from build123d import *

# Parameters (mm, degrees)
BOSS_EXTRUDE1_DEPTH     = 17.78
FILLET1_R               = 2
FILLET2_R               = 3
CUT_EXTRUDE5_DEPTH      = 34.999094106
CUT_EXTRUDE6_DEPTH      = 3
CUT_EXTRUDE7_DEPTH      = 3
CUT_EXTRUDE7_DEPTH_BACK = 1.5
BOSS_EXTRUDE2_DEPTH     = 8


with BuildPart() as part:
    # Sketch1 → Boss-Extrude1 (new body)
    with BuildSketch(Plane.XY):
        Polygon((0, 3), (0, 0), (7.3, 0), (7.3, 10), (13.3, 10), (19.3, 10), (19.3, 0), (26.6, 0), (26.6, 3), (20.8, 3), (20.8, 11.5), (5.8, 11.5), (5.8, 3), align=None)
    extrude(amount=-BOSS_EXTRUDE1_DEPTH)

    # Fillet1
    fillet1_edges = [part.edges().sort_by_distance(p)[0] for p in [
        (5.8, 11.5, -8.89),
        (20.8, 11.5, -8.89),
    ]]
    fillet(fillet1_edges, radius=FILLET1_R)

    # Fillet2
    fillet2_edges = [part.edges().sort_by_distance(p)[0] for p in [
        (5.8, 3, -8.89),
        (20.8, 3, -8.89),
    ]]
    fillet(fillet2_edges, radius=FILLET2_R)

    # Sketch2 → Cut-Extrude5 (cut, through all)
    with BuildSketch(Plane(origin=(0, 0, 0), x_dir=(1, 0, 0), z_dir=(0, 1, 0))):
        with BuildLine():
            Line((0, 17.78), (0, 4.65))
            ThreePointArc((0, 4.65), (1.361953467, 7.938046533), (4.65, 9.3))
            Line((4.65, 9.3), (4.65, 17.78))
            Line((4.65, 17.78), (0, 17.78))
        make_face()
        with BuildLine():
            Line((0, 4.65), (0, 0))
            Line((0, 0), (4.65, 0))
            ThreePointArc((4.65, 0), (1.361953467, 1.361953467), (0, 4.65))
        make_face()
        with BuildLine():
            ThreePointArc((21.95, 9.3), (25.238046535, 7.93804653), (26.6, 4.649999993))
            Line((26.6, 4.649999993), (26.6, 17.78))
            Line((26.6, 17.78), (21.95, 17.78))
            Line((21.95, 17.78), (21.95, 9.3))
        make_face()
        with BuildLine():
            Line((21.95, 0), (26.6, 0))
            Line((26.6, 0), (26.6, 4.649999993))
            ThreePointArc((26.6, 4.649999993), (25.23804653, 1.361953465), (21.95, 0))
        make_face()
    extrude(amount=CUT_EXTRUDE5_DEPTH, mode=Mode.SUBTRACT)

    # Sketch3 → Cut-Extrude6 (cut)
    with BuildSketch(Plane.XZ):
        with BuildLine():
            Line((7.3, -6.649999971), (7.3, -2.649999971))
            Line((7.3, -2.649999971), (5.8, -2.649999971))
            Line((5.8, -2.649999971), (5.8, -3.449999971))
            Line((5.8, -3.449999971), (4.6, -3.449999971))
            ThreePointArc((4.6, -3.449999971), (3.4, -4.649999971), (4.6, -5.849999971))
            Line((4.6, -5.849999971), (5.8, -5.849999971))
            Line((5.8, -5.849999971), (5.8, -6.649999971))
            Line((5.8, -6.649999971), (7.3, -6.649999971))
        make_face()
        with BuildLine():
            Line((20.8, -5.849999971), (22, -5.849999971))
            ThreePointArc((22, -5.849999971), (23.2, -4.649999971), (22, -3.449999971))
            Line((22, -3.449999971), (20.8, -3.449999971))
            Line((20.8, -3.449999971), (20.8, -2.649999971))
            Line((20.8, -2.649999971), (19.3, -2.649999971))
            Line((19.3, -2.649999971), (19.3, -6.649999971))
            Line((19.3, -6.649999971), (20.8, -6.649999971))
            Line((20.8, -6.649999971), (20.8, -5.849999971))
        make_face()
    extrude(amount=-CUT_EXTRUDE6_DEPTH, mode=Mode.SUBTRACT)

    # Sketch4 → Cut-Extrude7 (cut, two sides: drawn at the far end of the back side and taken through both)
    with BuildSketch(Plane(origin=(0, 3, 0), x_dir=(1, 0, 0), z_dir=(0, 1, 0)).offset(-CUT_EXTRUDE7_DEPTH_BACK)):
        Polygon((2.8, 3.189230456), (2.8, 6.110769486), (2.434936491, 5.899999971), (2.434936491, 3.399999971), align=None)
        Polygon((4.6, 2.149999971), (4.6, 4.649999971), (4.6, 7.149999971), (2.8, 6.110769486), (2.8, 3.189230456), align=None)
        Polygon((5.8, 2.842820294), (4.6, 2.149999971), (4.6, 4.649999971), (4.6, 7.149999971), (5.8, 6.457179648), align=None)
        Polygon((22, 2.149999971), (22, 4.649999971), (22, 7.149999971), (20.8, 6.457179648), (20.8, 2.842820294), align=None)
        Polygon((24.165063509, 5.899999971), (24.165063509, 3.399999971), (22, 2.149999971), (22, 4.649999971), (22, 7.149999971), align=None)
    extrude(amount=CUT_EXTRUDE7_DEPTH + CUT_EXTRUDE7_DEPTH_BACK, mode=Mode.SUBTRACT)

    # Sketch5 → Boss-Extrude2 (add)
    with BuildSketch(Plane(origin=(0, 0, 0), x_dir=(-1, 0, 0), z_dir=(0, 0, -1))):
        with BuildLine():
            Line((-16.3, 10), (-19.3, 10))
            Line((-19.3, 10), (-19.3, 7))
            ThreePointArc((-19.3, 7), (-18.421320344, 9.121320344), (-16.3, 10))
        make_face()
        with BuildLine():
            Line((-7.3, 7), (-7.3, 10))
            Line((-7.3, 10), (-10.3, 10))
            ThreePointArc((-10.3, 10), (-8.178679656, 9.121320344), (-7.3, 7))
        make_face()
    extrude(amount=BOSS_EXTRUDE2_DEPTH)


solid = part.part
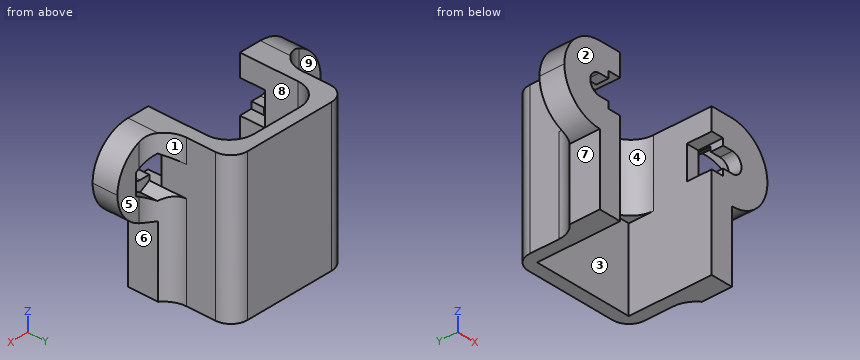
Read the model definition and answer for the solid it produces. Units are mm, in the model's axes. Face numbers are marked on the shaded views. A direction names the side the tool comes from. Coordinates: 2 decimals unless noted, no trailing zeros. Order: outer loops, then holes, each group sorted by start corner. A loop starts at its lowest first (then second) coordinate and runs counter-clockwise, first axis right, second up. Notation, with made-up numbers: M 31,81 L 58,81 A23 cw 58,112 Z; hole C -35.75,58.5 d10. An arc over 180 degrees is marked long. Put each result on its own line as item: value. Start each with the question number.
Item 1: Section B-B, the plane x = 8.5 is taken. Determine the outline of the cut face in (y, z), plus the area to 3 significant figures.
Item 2: Section A-A, the plane z = -10 is taken. Determine the outline of the cut face in (x, y), plus the area to 3 significant figures.
Item 3: Section C-C, the plane y = 7.5 is taken. Determine the outline of the cut face in (x, z).
Item 4: Consider probe 1 along X at (y, z) = (2.25, -13.5); probe 2 along Z at (x, y) = (19.5, 1.75); probe 3 along X at (y, z) = (9, -17). Determine where each line is inside the solid, lowest interval first. Write a range as [from, to].
Item 5: The mould has two halves that part along X. Classify the marked faces 1, 2, 3 and 4: +X half, -X half, draft (parallel to the pull), parting line (faces both ways), or undercut.
Item 6: Section D-D, the plane z = -1.75 is taken. Determine the outline of the cut face in (x, y), plus the area to 3 significant figures.
Item 7: Given pin 1 Ø0.9 at (y, z) = (1.5, -3) entering from +X; pin 2 Ø1.5 at (x, z) = (17.5, -6.5) entering from -Y; pin 3 Ø1.5 at (x, z) = (15.5, -6.5) entering from -Y, each flat-ended and moving along its own axis, determine where each tip first touches the part or whether it passes through.
Item 8: For the marked faces 5, 6, 7, 8 and 9, determine the directions among +Z, -Z, +X, -X, +Y, -Y from which every point of the face is accessible in a straight line to the end or side of a thin tool.
Computed:
1. outline: M 9.4,-8 L 10,-8 L 10,-17.78 L 11.5,-17.78 L 11.5,0 L 9.4,0 Z
1. area: 31.5 mm2
2. outline: M 4.65,0 L 7.3,0 L 7.3,10 L 19.3,10 L 19.3,0 L 21.95,0 L 21.95,3.64 A3 cw 20.8,6 L 20.8,9.5 A2 ccw 18.8,11.5 L 7.8,11.5 A2 ccw 5.8,9.5 L 5.8,6 A3 cw 4.65,3.64 Z
2. area: 60.8 mm2
3. outline: M 5.8,-17.78 L 7.3,-17.78 L 7.3,-8 L 7.34,-8 L 7.34,0 L 5.8,0 Z; M 19.26,-8 L 19.3,-8 L 19.3,-17.78 L 20.8,-17.78 L 20.8,0 L 19.26,0 Z
4. probe 1: x = [4.65, 7.3], [19.3, 21.95]
4. probe 2: z = [-17.78, -6.65], [-2.65, 0]
4. probe 3: x = [5.8, 7.3], [19.3, 20.8]
5. face 1: +X half
5. face 2: draft
5. face 3: undercut
5. face 4: undercut
6. outline: M 1.02,0 L 7.3,0 L 7.3,7 A3 cw 10.3,10 L 16.3,10 A3 cw 19.3,7 L 19.3,0 L 25.58,0 L 25.58,3 L 23.8,3 A3 cw 20.8,6 L 20.8,9.5 A2 ccw 18.8,11.5 L 7.8,11.5 A2 ccw 5.8,9.5 L 5.8,6 A3 cw 2.8,3 L 1.02,3 Z
6. area: 87.2 mm2
7. pin 1: stops at x = 26.44
7. pin 2: stops at y = 9.28
7. pin 3: stops at y = 10
8. face 5: +Z, -Z, +X, +Y
8. face 6: -Z, +X, +Y, -Y
8. face 7: -Z, -X, +Y, -Y
8. face 8: -Z, -Y
8. face 9: +Z, -Z, -X, +Y
